Drawing for the job (mm, zero at the part's lowest x, y, z). A direction names the side the tool comes from. Coordinates: 2 decimals unless noted, no trailing zeros. Order: outer loops, then holes, each group sorted by start corner. A loop starts at its lowest first (then second) coordinate and runs counter-clockwise, first axis right, second up. Notation, with made-up numbers: (-28.5, 15.25) -> (-17.5, 15.25) arc R31 cw to (-17.5, 49.25) -> close; hole circle Ø10 at (63, 82.5). An arc over 180 degrees is marked (long way). Write each question's results on one line, items separated by ' | '.
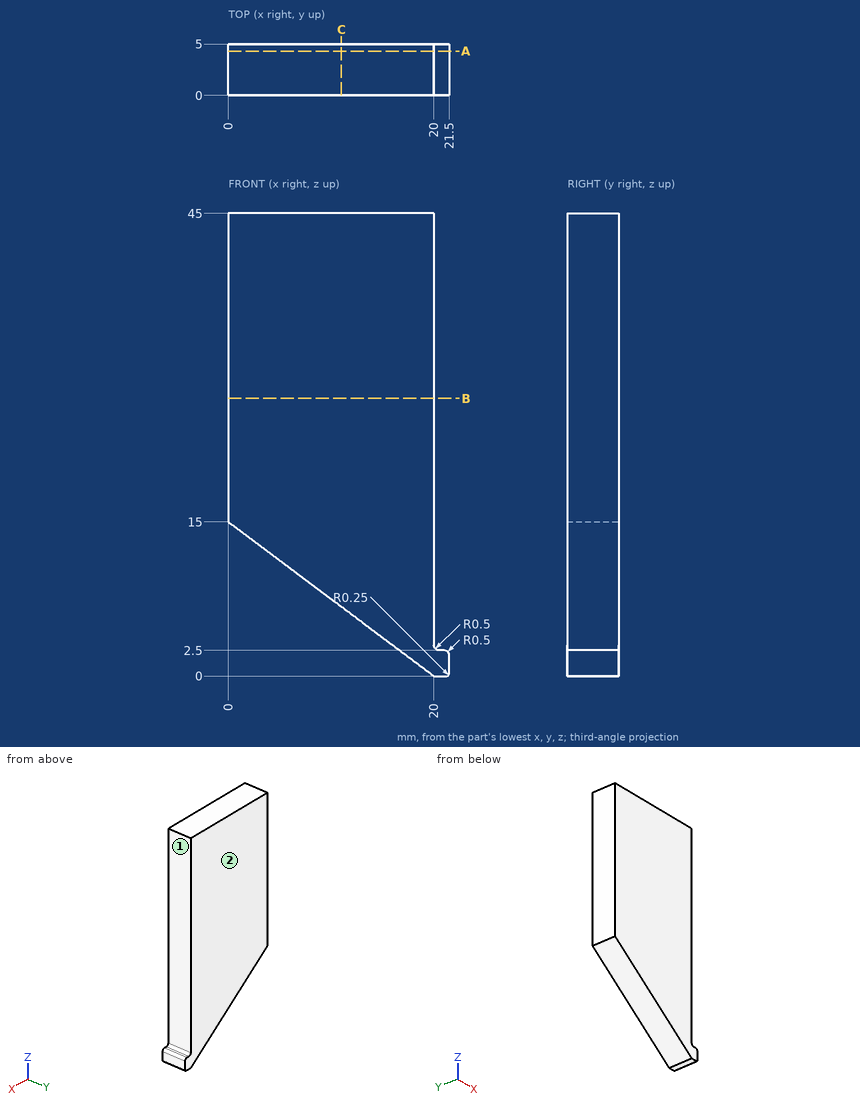
Item 1: Tool access for the marked faces 1 and 2: list every direction of +Z, -Z, +X, -X, +Y, -Y with a clear straight run to the whole face (end or side of a thin tool).
Answer:
face 1: +Z, +X, +Y, -Y | face 2: +Z, -Z, +X, -X, +Y
Item 2: Slice it at C-C, the plane x = 11. List the corners of the cut face in (y, z), and give its area (3 significant figures).
Answer:
outline: (0, 6.75) -> (5, 6.75) -> (5, 45) -> (0, 45) -> close | area: 191 mm^2
Item 3: Drill centre lines: line 1 (X direction, y = 2, z = 29); line 2 (X direction, y = 2.85, z = 8); line 3 (Z direction, x = 5.5, y = 4.1) (3 decimals). Where is each one in solid material? Low to high. Write a range as from..to.
Answer:
line 1: x = 0..20 | line 2: x = 9.33..20 | line 3: z = 10.875..45
Item 4: Slice it at A-A, the plane y = 4.3. List the corners of the cut face in (x, z).
Answer:
outline: (0, 15) -> (20, 0) -> (21.25, 0) arc R0.25 ccw to (21.5, 0.25) -> (21.5, 2) arc R0.5 ccw to (21, 2.5) -> (20.5, 2.5) arc R0.5 cw to (20, 3) -> (20, 45) -> (0, 45) -> close
Item 5: Pin check, flat tips, straight feed: pin 1 (2 mm diameter, centred on y = 1.5, z = 8.5, fed in from -X); pin 2 (2 mm diameter, centred on y = 1, z = 7.5, fed in from -X); pin 3 (2.5 mm diameter, centred on y = 1.5, z = 25.5, fed in from +X); pin 4 (3 mm diameter, centred on x = 8.5, z = 25, fed in from -Y). Stop position of each tip, or through.
Answer:
pin 1: stops at x = 7.33 | pin 2: stops at x = 8.67 | pin 3: stops at x = 20 | pin 4: stops at y = 0
Item 6: Slice it at B-B, the plane z = 27. List the corners of the cut face in (x, y).
Answer:
outline: (0, 0) -> (20, 0) -> (20, 5) -> (0, 5) -> close
